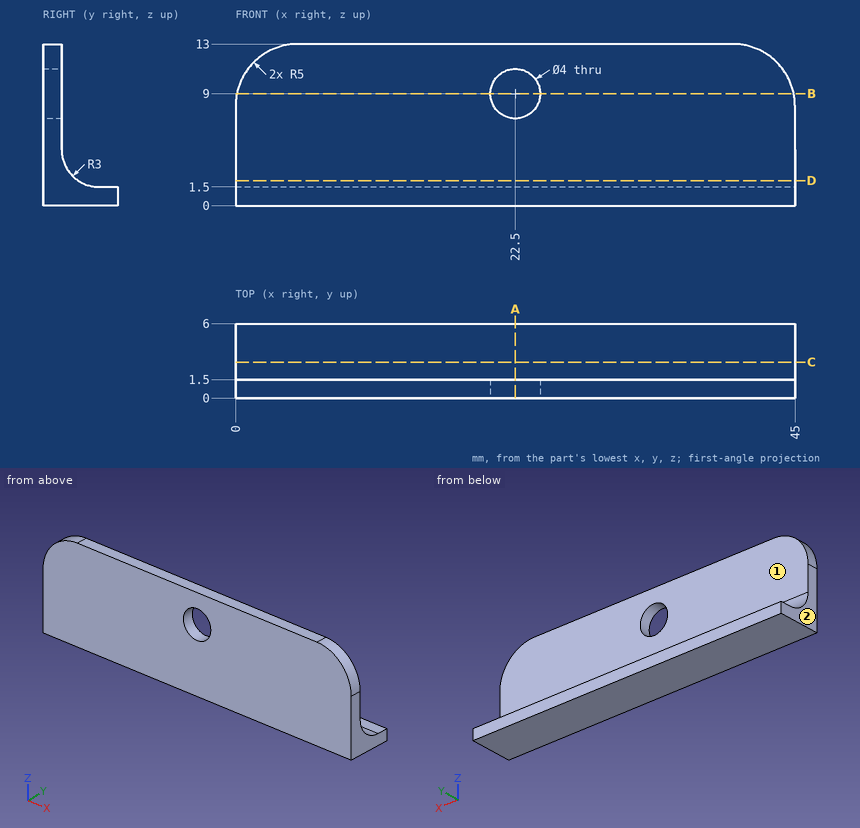
Geometry: see drawing. Coordinates: mm, zero at the bounding-box minimum. A direction names the side the tool comes from. Give positions to 0.01 mm unless a question says otherwise; leave off trailing zeros. Order: outer loops, then holes, each group sorted by start corner. A loop starts at its lowest first (then second) coordinate and runs counter-clockwise, first axis right, second up. Notation, with made-up numbers: (35, 73.25) - (72, 73.25) arc R13 ccw to (72, 86.25) - close; hole circle Ø4 at (-14, 38.5). An arc over 180 degrees is marked (long way). Write each question's results on one line, items separated by ' | '.
Item 1: Access query for the marked faces 1 and 2. Directions: +Z, -Z, +X, -X, +Y, -Y. A direction counts if a zero-diameter tool reaches every point of the face in a straight line with its end or side. Return the directions, or none.
A:
face 1: +Z, +X, -X, +Y | face 2: +Z, -Z, -X, +Y, -Y
Item 2: Section A-A (x = 22.5). Return loops of the section in (y, z).
A:
outline: (0, 0) - (6, 0) - (6, 1.5) - (4.5, 1.5) arc R3 cw to (1.5, 4.5) - (1.5, 7) - (0, 7) - close; (0, 11) - (1.5, 11) - (1.5, 13) - (0, 13) - close
Item 3: Section C-C (y = 2.9). Return loops of the section in (x, z).
A:
outline: (0, 0) - (45, 0) - (45, 1.96) - (0, 1.96) - close
Item 4: Section B-B (z = 9). Return loops of the section in (x, y).
A:
outline: (0.1, 0) - (20.5, 0) - (20.5, 1.5) - (0.1, 1.5) - close; (24.5, 0) - (44.9, 0) - (44.9, 1.5) - (24.5, 1.5) - close
Item 5: Section D-D (z = 2). Return loops of the section in (x, y), and give its area (3 significant figures).
A:
outline: (0, 0) - (45, 0) - (45, 2.84) - (0, 2.84) - close | area: 128 mm^2
Item 6: Contact query for flat-ended pins moving along their axis: pin 1 Ø2 at (y, z) = (1, 10) entering from +X; pin 2 Ø3.5 at (x, z) = (22.5, 9) entering from -Y; pin 3 Ø4.5 at (x, z) = (32, 7) entering from +Y. Output: stop coordinate, or through.
A:
pin 1: stops at x = 44.9 | pin 2: passes through | pin 3: stops at y = 1.5
Item 7: Material intervals for line 1 along Z through (x, y) = (29, 5.45); line 2 along X through (y, z) = (0.45, 9), sorted ascending.
A:
line 1: z = 0 to 1.5 | line 2: x = 0.1 to 20.5, 24.5 to 44.9
